Geometry check sheet. Reference: the model listing, model coordinates, mm. Face numbers are marked on the shaded views. Round coordinates to 2 decimals unless told otherwise and drop trailing zeros. Write each loop counter-clockwise with the first axis right and the second up, starting at its lowest first coordinate (ties: lowest second). Pieces come first, ordered by that corner, then holes. Notation, with made-up numbers: (-32, -31) -> (24, -31) arc R11 ccw to (24, -13) -> close; hole circle Ø4 at (81, 58.5). An arc over 180 degrees is marked (long way). Use a Markdown table: item, result.
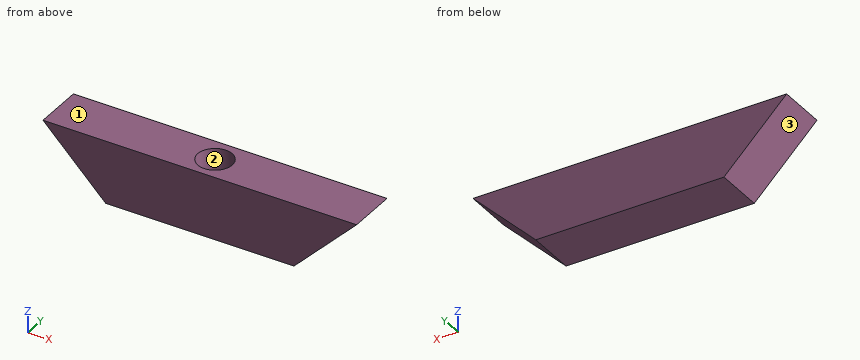
```python
from build123d import *

# Parameters (mm, degrees)
F1_DEPTH = 3.9
F3_D     = 5.5
F3_DEPTH = 8
F3_TIP   = 1.6523667023


with BuildPart() as f1:
    # F0 (on Front) → F1 (new body, symmetric)
    with BuildSketch(Plane.XZ):
        Polygon((-25, 10), (-15, 0), (15, 0), (25, 10), align=None)
    extrude(amount=F1_DEPTH, both=True)

    # F3
    with Locations(Plane.XY.offset(10)):
        with Locations((0, 0)):
            Hole(F3_D / 2, depth=F3_DEPTH)
            with Locations((0, 0, -(F3_DEPTH + F3_TIP / 2))):  # 118° drill point
                Cone(0, F3_D / 2, F3_TIP, mode=Mode.SUBTRACT)


solid = f1.part
```
(1) Section check D-D on x = -21. Record the cut outline in (y, z), plus the area to 3 significant figures.
A:
| item | result |
|---|---|
| outline | (-3.9, 6) -> (3.9, 6) -> (3.9, 10) -> (-3.9, 10) -> close |
| area | 31.2 mm2 |
(2) Section check A-A on z = 4.25. Record the cut outline in (x, y).
A:
| item | result |
|---|---|
| outline | (-19.25, -3.9) -> (19.25, -3.9) -> (19.25, 3.9) -> (-19.25, 3.9) -> close; hole circle Ø5.5 at (0, 0) |
(3) Thickness scan on line 1 (Y direction, x = 0, z = 6.5); line 2 (X direction, y = 0, z = 6); line 3 (X direction, y = 0, z = 5). Record the ranges inside material, lowest first.
A:
| item | result |
|---|---|
| line 1 | y = -3.9 to -2.75, 2.75 to 3.9 |
| line 2 | x = -21 to -2.75, 2.75 to 21 |
| line 3 | x = -20 to -2.75, 2.75 to 20 |
(4) Section check B-B on y = 3.25. Record the cut outline in (x, z).
A:
| item | result |
|---|---|
| outline | (-25, 10) -> (-15, 0) -> (15, 0) -> (25, 10) -> close |
(5) Gauge pin test, flat ends, axial feed: pin 1 Ø1.5 at (y, z) = (1.5, 2) entering from -X; pin 2 Ø2 at (y, z) = (-2.5, 3) entering from -X; pin 3 Ø1 at (x, y) = (-18, 2) entering from -Z. Record the tip position at first contact, or that the pin passes through.
A:
| item | result |
|---|---|
| pin 1 | stops at x = -17.75 |
| pin 2 | stops at x = -19 |
| pin 3 | stops at z = 2.5 |
(6) Release check for a two-part mould opening along X. For the marked faces 1, 2 and 3 record: +X half, -X half, draft (parallel to the pull), parting line (faces both ways), or undercut.
A:
| item | result |
|---|---|
| face 1 | draft |
| face 2 | undercut |
| face 3 | -X half |
(7) Section check C-C on z = 8.75. Record the cut outline in (x, y).
A:
| item | result |
|---|---|
| outline | (-23.75, -3.9) -> (23.75, -3.9) -> (23.75, 3.9) -> (-23.75, 3.9) -> close; hole circle Ø5.5 at (0, 0) |
